Read the model definition and answer for the solid it produces. Units are mm, in the model's axes. Face numbers are marked on the shaded views. A direction names the side the tool comes from. Coordinates: 2 decimals unless noted, no trailing zeros. Order: outer loops, then holes, each group sorted by start corner. A loop starts at its lowest first (then second) coordinate and runs counter-clockwise, first axis right, second up.
```python
from build123d import *

# Parameters (mm, degrees)
SKETCH1_R           = 7.5
BOSS_EXTRUDE1_DEPTH = 10
SKETCH1_3_W         = 50
SKETCH1_3_H         = 10
BOSS_EXTRUDE2_DEPTH = 75
CUT_EXTRUDE1_REACH  = 142.847


with BuildPart() as part:
    # Sketch1 → Boss-Extrude1 (new body)
    with BuildSketch(Plane(origin=(0, 0, 0), x_dir=(1, 0, 0), z_dir=(0, 1, 0))):
        with BuildLine():
            Line((25, 0), (-25, 0))
            Line((-25, 0), (-25, -17.151864589))
            ThreePointArc((-25, -17.151864589), (-25.701702665, -20.83176495), (-27.708333333, -23.995226133))
            ThreePointArc((-27.708333333, -23.995226133), (-37.256095308, -42.517796957), (-35.600057015, -63.29044546))
            Line((-35.600057015, -63.29044546), (-22.848639927, -57.34436202))
            ThreePointArc((-22.848639927, -57.34436202), (21.751386889, -39.857161718), (-20.312930357, -62.782208742))
            Line((-20.312930357, -62.782208742), (-33.064347445, -68.728292182))
            ThreePointArc((-33.064347445, -68.728292182), (-31.119955968, -71.807070885), (-28.889805354, -74.685606061))
            ThreePointArc((-28.889805354, -74.685606061), (-21.739686255, -85.712027428), (-17.709540124, -98.220588235))
            ThreePointArc((-17.709540124, -98.220588235), (0, -113), (17.709540124, -98.220588235))
            ThreePointArc((17.709540124, -98.220588235), (21.739686255, -85.712027428), (28.889805354, -74.685606061))
            ThreePointArc((28.889805354, -74.685606061), (37.989682547, -49.114550984), (27.708333333, -23.995226133))
            ThreePointArc((27.708333333, -23.995226133), (25.701702665, -20.83176495), (25, -17.151864589))
            Line((25, -17.151864589), (25, 0))
        make_face()
        with Locations(Location((0, -95, 0), (0, 0, 270))):
            Circle(SKETCH1_R, mode=Mode.SUBTRACT)
    extrude(amount=BOSS_EXTRUDE1_DEPTH)

    # Sketch1_3 → Boss-Extrude2 (add)
    with BuildSketch(Plane(origin=(0, 0, 0), x_dir=(1, 0, 0), z_dir=(0, 1, 0))):
        with Locations((0, 5)):
            Rectangle(SKETCH1_3_W, SKETCH1_3_H)
    extrude(amount=BOSS_EXTRUDE2_DEPTH)

    # Sketch2 → Cut-Extrude1 (cut, up to next)
    with BuildSketch(Plane.XY, mode=Mode.PRIVATE) as cut_extrude1_sk1:
        with BuildLine():
            Line((-7, 50), (-7, 25))
            ThreePointArc((-7, 25), (0, 18), (7, 25))
            Line((7, 25), (7, 50))
            ThreePointArc((7, 50), (0, 57), (-7, 50))
        make_face()
    cut_extrude1_tool1 = extrude(cut_extrude1_sk1.sketch, amount=-CUT_EXTRUDE1_REACH, mode=Mode.PRIVATE) & part.part
    # Sketch2 → Cut-Extrude1 (cut, up to next)
    with BuildSketch(Plane.XY, mode=Mode.PRIVATE) as cut_extrude1_sk2:
        with BuildLine():
            ThreePointArc((2.6e-08, 75), (17.677669539, 67.67766952), (25, 50))
            Line((25, 50), (25, 75))
            Line((25, 75), (2.6e-08, 75))
        make_face()
    cut_extrude1_tool2 = extrude(cut_extrude1_sk2.sketch, amount=-CUT_EXTRUDE1_REACH, mode=Mode.PRIVATE) & part.part
    # Sketch2 → Cut-Extrude1 (cut, up to next)
    with BuildSketch(Plane.XY, mode=Mode.PRIVATE) as cut_extrude1_sk3:
        with BuildLine():
            ThreePointArc((-25, 50), (-17.67766952, 67.677669539), (2.6e-08, 75))
            Line((2.6e-08, 75), (-25, 75))
            Line((-25, 75), (-25, 50))
        make_face()
    cut_extrude1_tool3 = extrude(cut_extrude1_sk3.sketch, amount=-CUT_EXTRUDE1_REACH, mode=Mode.PRIVATE) & part.part
    add(cut_extrude1_tool1.solids().sort_by_distance((0, 37.5, 0))[0], mode=Mode.SUBTRACT)
    add(cut_extrude1_tool2.solids().sort_by_distance((19.415802, 69.415802, 0))[0], mode=Mode.SUBTRACT)
    add(cut_extrude1_tool3.solids().sort_by_distance((-19.415802, 69.415802, 0))[0], mode=Mode.SUBTRACT)


solid = part.part
```
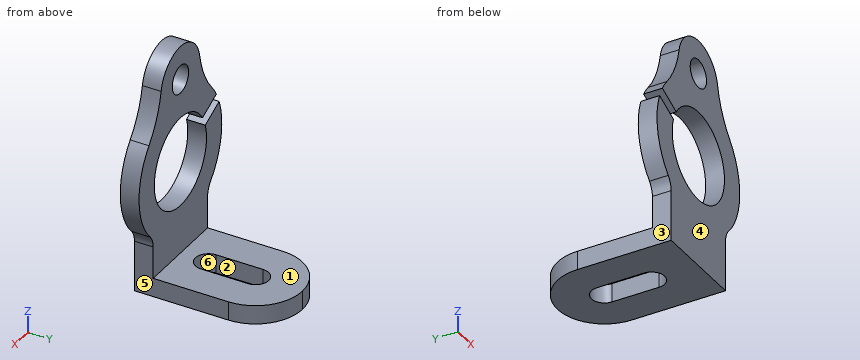
1) A cutting plane is placed at A-A, the plane z = 50. Determine the outline of the cut face in (x, y).
A:
outline: (-38, 0) - (-24, 0) - (-24, 10) - (-38, 10) - close; (24, 0) - (38, 0) - (38, 10) - (24, 10) - close
2) Straight lines are drawn through the part: line 1 (X direction, y = 3, z = 50); line 2 (Y direction, x = -27.5, z = 50); line 3 (X direction, y = 5.5, z = 0.5). For each, find the intervals that lie inside material, in ascending order.
A:
line 1: x = -38 to -24, 24 to 38
line 2: y = 0 to 10
line 3: x = -25 to 25
3) A cutting plane is placed at D-D, the plane z = 7.5. Determine the outline of the cut face in (x, y).
A:
outline: (-25, 0) - (25, 0) - (25, 10) - (-25, 10) - close
4) A cutting plane is placed at B-B, the plane y = 43. Determine the outline of the cut face in (x, z), and give its area (3 significant figures).
A:
outline: (-25, -10) - (-7, -10) - (-7, 0) - (-25, 0) - close; (7, -10) - (25, -10) - (25, 0) - (7, 0) - close
area: 360 mm2
5) Which of the six approach directions +Z, -Z, +X, -X, +Y, -Y give full straight-line access (tool end or side, diameter ignored) to the marked faces 1, 2 and 3?
A:
face 1: +Z, +X, -X, +Y
face 2: +Z, -Z
face 3: -Z, -X, +Y, -Y
6) A cutting plane is placed at C-C, the plane x = 21.5. Determine the outline of the cut face in (y, z), and give its area (3 significant figures).
A:
outline: (0, -10) - (62.76, -10) - (62.76, 0) - (10, 0) - (10, 39.33) - (0, 39.33) - close; (0, 60.67) - (10, 60.67) - (10, 86.22) - (0, 86.22) - close
area: 1,280 mm2
7) Determine the mould class of the marked faces 4, 5 and 6 for opening direction X: pulls with the +X half, pulls with the -X half, needs draft (parallel to the pull), parting line crosses it, or undercut.
A:
face 4: needs draft
face 5: pulls with the +X half
face 6: undercut
8) Flat-ended cylindrical pins translate along their axes: pin 1 Ø1.5 at (x, y) = (24, 28.5) entering from +Z; pin 2 Ø3 at (y, z) = (43, -3.5) entering from +X; pin 3 Ø11 at (y, z) = (35.5, -3) entering from -X. Find the tip coordinate at first contact, or state that the pin passes through.
A:
pin 1: stops at z = 0
pin 2: stops at x = 25
pin 3: stops at x = -25
